For this review, take the finished solid that the model builds, in its own axes (mm). A direction names the side the tool comes from. Round coordinates to 2 decimals unless told otherwise and drop trailing zeros. Order: outer loops, then holes, each group sorted by start corner. A loop starts at its lowest first (then second) coordinate and runs counter-clockwise, first axis right, second up. Notation, with made-up numbers: (-31, -1) -> (-3, -1) arc R19 cw to (-3, 27) -> close; hole circle Ø10 at (-13.5, 3). An arc over 180 degrees is marked (long way). Use a Markdown table: item, result. Add a question column.
1) Machinability: for faces 1 (the face through (0.66, 86.781, -14.985)), 2 (the face through (0, -204.756, 0)), 3 (the face through (-39.923, -112.668, 20.765)), which of the approach directions +Z, -Z, +X, -X, +Y, -Y give a long, thin tool a straight path to every point of the face, cutting with its end or side? Answer none if there is none.
2) Clearance check with flat-ended pins moving along their axes: P1, Ø1.5, axis at x = -36, z = -30, coming from the -Y side; P2, Ø1, axis at y = -21.5, z = 11, coming from the +X side; P3, Ø1, axis at x = 6, y = -59, coming from the +Z side. State where each tip first meets the part, or that it passes through.
3) Consider section A-A (y = 31). State the section outline as (x, z) points.
4) Consider section B-B (y = -143). State the section outline as (x, z) points.
5) Wall thickness on line 1 along X through (y, z) = (-85.5, 0); line 2 along Y through (x, z) = (36.5, 5); line 3 along Y through (x, z) = (-27, -25): over which ranges is each line inside the solid? List them lowest first. Write a range as [from, to].
```python
from build123d import *


with BuildPart() as f1:
    # F0 (on Right) → F1 (revolve)
    with BuildSketch(Plane.YZ):
        with BuildLine():
            Line((-204.756087, 20), (-204.756087, 0))
            Line((-204.756087, 0), (95.243913, 0))
            Line((95.243913, 0), (95.243913, 15))
            Line((95.243913, 15), (78.551713, 15))
            ThreePointArc((78.551713, 15), (71.480645, 17.928932), (68.551713, 25))
            Line((68.551713, 25), (68.551713, 26.717782))
            ThreePointArc((68.551713, 26.717782), (62.693848, 40.859917), (48.551713, 46.717782))
            Line((48.551713, 46.717782), (-11.037248, 46.717782))
            ThreePointArc((-11.037248, 46.717782), (-26.568814, 30.899643), (-43.675041, 45))
            Line((-43.675041, 45), (-179.756087, 45))
            ThreePointArc((-179.756087, 45), (-197.433757, 37.67767), (-204.756087, 20))
        make_face()
    revolve(axis=Axis((0, -4.756087, 0), (0, 1, 0)))


solid = f1.part
```
Results list:
| question | item | result |
|---|---|---|
| 1 | face 1 | +Y |
| 1 | face 2 | +Z, -Z, +X, -X, -Y |
| 1 | face 3 | -Y |
| 2 | P1 | y = -11.07 |
| 2 | P2 | x = 30.32 |
| 2 | P3 | z = 44.66 |
| 3 | outline | circle Ø93.44 at (0, 0) |
| 4 | outline | circle Ø90 at (0, 0) |
| 5 | line 1 | [-45, 45] |
| 5 | line 2 | [-198.23, -40.08], [-14.78, 65.8] |
| 5 | line 3 | [-198.27, -40.05], [-14.81, 65.83] |
